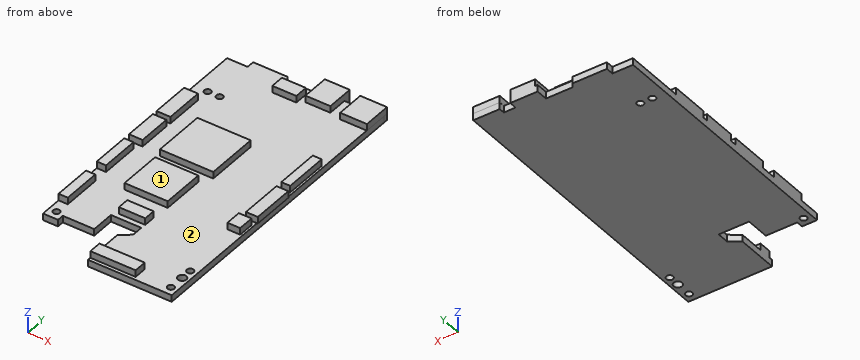
```python
from build123d import *

# Parameters (mm, degrees)
BOSS_EXTRU_1_DEPTH  = 2
ESQUISSE3_W         = 15.79325035
ESQUISSE3_H         = 15.667907094
BOSS_EXTRU_3_DEPTH  = 2
ESQUISSE4_W         = 12.785012189
ESQUISSE4_H         = 12.785012188
BOSS_EXTRU_4_DEPTH  = 2
ESQUISSE5_W         = 7.91948101
ESQUISSE5_H         = 8.397998202
BOSS_EXTRU_5_DEPTH  = 2
ESQUISSE6_W         = 7.37870607
ESQUISSE6_H         = 8.10533589
BOSS_EXTRU_6_DEPTH  = 2
ESQUISSE7_W         = 2.632934746
ESQUISSE7_H         = 13.164673727
ESQUISSE7_W_2       = 3.510579661
ESQUISSE7_H_2       = 12.788540192
ESQUISSE7_W_3       = 3.761335351
ESQUISSE7_H_3       = 4.764358111
ESQUISSE7_W_4       = 7.8
ESQUISSE7_H_4       = 3.5
ESQUISSE7_W_5       = 13.4
ESQUISSE7_H_5       = 3.8
ESQUISSE7_W_6       = 2.742200186
ESQUISSE7_H_6       = 11.5
ESQUISSE7_W_7       = 4
ESQUISSE7_H_7       = 10
ESQUISSE7_W_8       = 7.11
ESQUISSE7_H_8       = 4
ESQUISSE7_W_9       = 4.11
ESQUISSE7_H_9       = 11.55
BOSS_EXTRU_7_DEPTH  = 2
SKETCH_3_R          = 1
SKETCH_3_R_2        = 1.25
CUT_EXTRUDE_4_DEPTH = 10
SKETCH_1_R          = 1
CUT_EXTRUDE_5_DEPTH = 10
SKETCH_2_R          = 1
CUT_EXTRUDE_6_DEPTH = 10


with BuildPart() as part:
    # Esquisse1 → Boss.-Extru.1 (new body)
    with BuildSketch(Plane.XY):
        Polygon((778.796370306, 167.014727296), (753.996370306, 167.014727296), (753.996370306, 179.284727296), (757.046370306, 181.630881142), (757.046370306, 185.030881142), (748.046370306, 185.030881142), (748.046370306, 178.030881142), (738.734755108, 178.030881142), (738.734755108, 176.030881142), (734.296370306, 176.030881142), (734.296370306, 253.030881142), (740.392724327, 253.030881142), (740.392724327, 255.330881142), (750.563009525, 255.330881142), (751.563009525, 254.030881142), (759.363009525, 254.030881142), (759.363009525, 257.573130323), (759.380880171, 257.573130323), (759.380880171, 257.530881142), (767.454666434, 257.530881142), (767.454666434, 255.306621268), (770.951996508, 255.306621268), (770.951996508, 257.014727296), (778.78419371, 257.014727296), (778.78419371, 255.894727296), (778.796370306, 255.894727296), align=None)
    extrude(amount=BOSS_EXTRU_1_DEPTH)

    # Esquisse3 → Boss.-Extru.3 (add)
    with BuildSketch(Plane(origin=(0, 0, 2), x_dir=(-1, 0, 0), z_dir=(0, 0, -1))):
        with Locations((-751.834833735, 219.169546492)):
            Rectangle(ESQUISSE3_W, ESQUISSE3_H)
    extrude(amount=-BOSS_EXTRU_3_DEPTH)

    # Esquisse4 → Boss.-Extru.4 (add)
    with BuildSketch(Plane(origin=(0, 0, 2), x_dir=(-1, 0, 0), z_dir=(0, 0, -1))):
        with Locations((-751.208117452, 201.684162176)):
            Rectangle(ESQUISSE4_W, ESQUISSE4_H)
    extrude(amount=-BOSS_EXTRU_4_DEPTH)

    # Esquisse5 → Boss.-Extru.5 (add)
    with BuildSketch(Plane(origin=(0, 0, 2), x_dir=(-1, 0, 0), z_dir=(0, 0, -1))):
        with Locations((-774.900958926, 252.812156779)):
            Rectangle(ESQUISSE5_W, ESQUISSE5_H)
    extrude(amount=-BOSS_EXTRU_5_DEPTH)

    # Esquisse6 → Boss.-Extru.6 (add)
    with BuildSketch(Plane(origin=(0, 0, 2), x_dir=(-1, 0, 0), z_dir=(0, 0, -1))):
        with Locations((-763.765313399, 253.478213197)):
            Rectangle(ESQUISSE6_W, ESQUISSE6_H)
    extrude(amount=-BOSS_EXTRU_6_DEPTH)

    # Esquisse7 → Boss.-Extru.7 (add)
    with BuildSketch(Plane(origin=(0, 0, 2), x_dir=(-1, 0, 0), z_dir=(0, 0, -1))):
        with Locations((-776.846036285, 224.074096482)):
            Rectangle(ESQUISSE7_W, ESQUISSE7_H)
        with Locations((-777.284858743, 209.091444002)):
            Rectangle(ESQUISSE7_W_2, ESQUISSE7_H_2)
        with Locations((-776.281835983, 198.935838556)):
            Rectangle(ESQUISSE7_W_3, ESQUISSE7_H_3)
        with Locations((-753.246370306, 188.280881142)):
            Rectangle(ESQUISSE7_W_4, ESQUISSE7_H_4)
        with Locations((-760.696370306, 169.914727296)):
            Rectangle(ESQUISSE7_W_5, ESQUISSE7_H_5)
        with Locations((-735.667470399, 188.280881142)):
            Rectangle(ESQUISSE7_W_6, ESQUISSE7_H_6)
        with Locations((-735.667470399, 204.280881142)):
            Rectangle(ESQUISSE7_W_6, ESQUISSE7_H_6)
        with Locations((-736.296370306, 217.030881142)):
            Rectangle(ESQUISSE7_W_7, ESQUISSE7_H_7)
        with Locations((-754.808009525, 250.030881142)):
            Rectangle(ESQUISSE7_W_8, ESQUISSE7_H_8)
        with Locations((-736.351370306, 229.305881142)):
            Rectangle(ESQUISSE7_W_9, ESQUISSE7_H_9)
    extrude(amount=-BOSS_EXTRU_7_DEPTH)

    # Эскиз3 → Вырез-Вытянуть4 (cut)
    with BuildSketch(Plane.XY.offset(2)):
        with Locations((738.296370306, 239.280881142)):
            Circle(SKETCH_3_R)
        with Locations((741.846370306, 239.280881142)):
            Circle(SKETCH_3_R)
        with Locations((776.796370306, 174.214727296)):
            Circle(SKETCH_3_R_2)
        with Locations((776.796370306, 177.614727296)):
            Circle(SKETCH_3_R)
    extrude(amount=-CUT_EXTRUDE_4_DEPTH, mode=Mode.SUBTRACT)

    # Эскиз1 → Вырез-Вытянуть5 (cut)
    with BuildSketch(Plane.XY.offset(2)):
        with Locations((736.515562707, 178.530881142)):
            Circle(SKETCH_1_R)
    extrude(amount=-CUT_EXTRUDE_5_DEPTH, mode=Mode.SUBTRACT)

    # Эскиз2 → Вырез-Вытянуть6 (cut)
    with BuildSketch(Plane.XY.offset(2)):
        with Locations((776.796370306, 169.514727296)):
            Circle(SKETCH_2_R)
    extrude(amount=-CUT_EXTRUDE_6_DEPTH, mode=Mode.SUBTRACT)


solid = part.part
```
Can you work these out from the model? Positions are in its coordinate system, mm. Face numbers are marked on the shaded views. Coordinates: 2 decimals unless noted, no trailing zeros. Loops run counter-clockwise (first coordinate to the right, second up) from the corner with the lowest first, then second, coordinate; pieces in that order, holes last.
Item 1: Suppose I cut it at D-D (y = 236). Please give me the cut outline in (x, z).
Answers below:
outline: (734.3, 0) - (778.8, 0) - (778.8, 2) - (734.3, 2) - close
Item 2: Please list where these lines run through material, in increasing order: L1, parallel to X at y = 207, z = 2.15; L2, parallel to X at y = 202, z = 2.3; L3, parallel to X at y = 174, z = 0.3.
Answers below:
L1: x = 734.3 to 737.04, 744.82 to 757.6, 775.53 to 779.04
L2: x = 734.3 to 737.04, 744.82 to 757.6
L3: x = 754 to 775.56, 778.03 to 778.8
Item 3: Suppose I cut it at A-A (y = 180.5). Please give me the cut outline in (x, z).
Answers below:
outline: (734.3, 0) - (748.05, 0) - (748.05, 2) - (734.3, 2) - close; (755.58, 0) - (778.8, 0) - (778.8, 2) - (755.58, 2) - close
Item 4: Suppose I cut it at B-B (x = 752.5). Please give me the cut outline in (y, z).
Answers below:
outline: (185.03, 0) - (254.03, 0) - (254.03, 2) - (252.03, 2) - (252.03, 4) - (248.03, 4) - (248.03, 2) - (227, 2) - (227, 4) - (211.34, 4) - (211.34, 2) - (208.08, 2) - (208.08, 4) - (195.29, 4) - (195.29, 2) - (190.03, 2) - (190.03, 4) - (186.53, 4) - (186.53, 2) - (185.03, 2) - close
Item 5: Suppose I cut it at C-C (z = 3.35). State how many separate pieces and enclosed holes the cut face has, then the cut area to 3 significant figures.
Answers below:
separate pieces: 14
enclosed holes: 0
area: 892 mm2
Item 6: I'm going to push flat-ended pins straight in: pin 1 (2 mm diameter, centred on x = 737, z = 3.5, fed in from +Y); pin 2 (1 mm diameter, centred on x = 749.5, y = 240.5, fed in from +Z); pin 3 (2 mm diameter, centred on x = 735.5, z = 3.5, fed in from -Y). Where does each tip first touch, or does it pass through?
Answers below:
pin 1: stops at y = 235.08
pin 2: stops at z = 2
pin 3: stops at y = 182.53
Item 7: If we mould it in two halves opening along X, with no side actions, what happens to the marked faces 1 and 2? For each: released by +X, released by -X, zero draft, split by the parting line, or undercut.
Answers below:
face 1: zero draft
face 2: undercut
